Design review of the part shown in the three views and the two pictorial views. Dimensions are in mm from the part's minimum x, y and z. A direction names the side the tool comes from. Coordinates: 2 decimals unless noted, no trailing zeros. Loops run counter-clockwise (first coordinate to the right, second up) from the corner with the lowest first, then second, coordinate; pieces in that order, holes last. Notation, with made-up numbers: (-39.5, 63) -> (3.5, 63) arc R28 cw to (3.5, 90) -> close; hole circle Ø8 at (73.5, -32.5). An arc over 180 degrees is marked (long way). Answer in a Markdown table with one row per item.
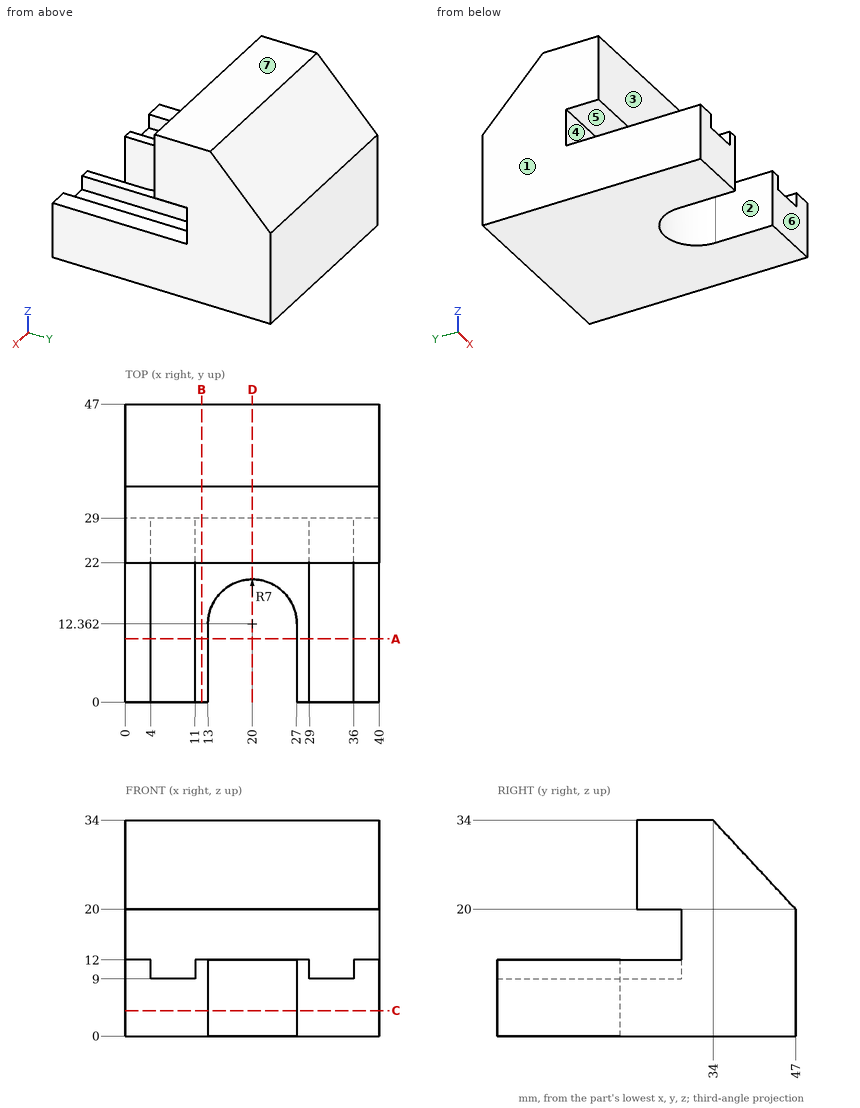
Item 1: For the marked faces 1, 2 and 3, list the 3-axis set-ups (+Z, -Z, +X, -X, +Y, -Y) from which the entire face can be reached by the end or side of a thin tool; tool diameter is ignored.
Worked answers:
| item | result |
|---|---|
| face 1 | +Z, -Z, -X, +Y, -Y |
| face 2 | +Z, -Z, -Y |
| face 3 | +Z, +X, -X, -Y |
Item 2: Take a section at B-B, the plane x = 12. State the section outline as (y, z) points.
Worked answers:
| item | result |
|---|---|
| outline | (0, 0) -> (47, 0) -> (47, 20) -> (34, 34) -> (22, 34) -> (22, 20) -> (29, 20) -> (29, 12) -> (0, 12) -> close |
Item 3: Insertion check: pin 1 (1.2 mm diameter, centred on x = 3, y = 14.5, fed in from +Z); pin 2 (5.5 mm diameter, centred on x = 32, y = 8.5, fed in from +Z); pin 3 (11 mm diameter, centred on x = 19, z = 30, fed in from -Y). Each pin has a flat end and moves straight along its axis. Give the tip position at first contact, or say it passes through.
Worked answers:
| item | result |
|---|---|
| pin 1 | z = 12 |
| pin 2 | z = 9 |
| pin 3 | y = 22 |
Item 4: The part is to be moulded in two halves that separate along Z. For the marked faces 4, 5, 6 and 7, say which applies: +Z half, -Z half, draft (parallel to the pull), parting line (faces both ways), or undercut.
Worked answers:
| item | result |
|---|---|
| face 4 | undercut |
| face 5 | undercut |
| face 6 | draft |
| face 7 | +Z half |
Item 5: Take a section at C-C, the plane z = 4. State the section outline as (x, y) points.
Worked answers:
| item | result |
|---|---|
| outline | (0, 0) -> (13, 0) -> (13, 12.36) arc R7 cw to (27, 12.36) -> (27, 0) -> (40, 0) -> (40, 47) -> (0, 47) -> close |
Item 6: Take a section at A-A, the plane y = 10. State the section outline as (x, z) points.
Worked answers:
| item | result |
|---|---|
| outline | (0, 0) -> (13, 0) -> (13, 12) -> (11, 12) -> (11, 9) -> (4, 9) -> (4, 12) -> (0, 12) -> close; (27, 0) -> (40, 0) -> (40, 12) -> (36, 12) -> (36, 9) -> (29, 9) -> (29, 12) -> (27, 12) -> close |
Item 7: For L1, parallel to Z at x = 17, y = 19; L2, parallel to X at y = 15.5, z = 4; L3, parallel to Y at x = 32, z = 14.5, list the stretches that pass through material, from the lowest coordinate up.
Worked answers:
| item | result |
|---|---|
| L1 | 0 to 12 |
| L2 | 0 to 13.74, 26.26 to 40 |
| L3 | 29 to 47 |
Item 8: Take a section at D-D, the plane x = 20. State the section outline as (y, z) points.
Worked answers:
| item | result |
|---|---|
| outline | (19.36, 0) -> (47, 0) -> (47, 20) -> (34, 34) -> (22, 34) -> (22, 20) -> (29, 20) -> (29, 12) -> (19.36, 12) -> close |
